Model file for the job. Use its own axes, mm. A direction names the side the tool comes from. Coordinates: 2 decimals unless noted, no trailing zeros. Write each loop counter-clockwise with the first axis right and the second up, starting at its lowest first coordinate (ties: lowest second). Pieces come first, ordered by that corner, then holes. Notation, with made-up numbers: (6.5, -23.75) - (51.5, -23.75) arc R19 cw to (51.5, -7.75) - close; hole circle Ø9 at (46, 34.25). An arc over 180 degrees is marked (long way). Put each result on its own line as item: value. Start each with the question number.
1. Saw through at B-B, the plane z = -21. Write the cut outline in (x, y) (3 decimals), plus the area to 3 significant figures.
2. Which spindle directions (+Z, -Z, +X, -X, +Y, -Y) get a long thin tool onto all of the face, cutting with end or side? Do faces 1 (the face through (9.855, 11.339, -1.565)), 2 (the face through (3.175, 19, -26)). Say none if no direction does.
3. Pull direction Y, two halves, no side cores. Call faces 3 (the face through (2, 19, -47.625)), 4 (the face through (23, 38.1, -18)), 5 (the face through (11.687, 31.793, -1.565)): released by +Y, released by -Y, zero draft, split by the parting line, or undercut.
4. Drop flat-ended pins along their axis: P1, Ø5.5, axis at x = 9.5, y = 20.5, coming from the -Z side (3 decimals); P2, Ø4, axis at y = 14.5, z = -10.5, coming from the -X side. Give the stop position or say it passes through.
5. Drill centre lines: L1, parallel to Y at x = 12.7, z = -1.1; L2, parallel to X at y = 21.5, z = -15 (3 decimals); L3, parallel to Y at x = 24.5, z = -38.1. Where is each one in solid material? Low to high. Write a range as from..to.
6. Saw through at C-C, the plane z = -38.1. Write the cut outline in (x, y) (3 decimals), plus the area to 3 significant figures.
7. Saw through at D-D, the plane y = 18.5. Write the cut outline in (x, z) (3 decimals).
8. Saw through at A-A, the plane x = 12.7. Write the cut outline in (y, z) (3 decimals), plus the area to 3 significant figures.
Autodesk Inventor part; units mm, degrees
ref_plane "YZ Plane" through (0, 0, 0) normal (1, 0, 0) x (0, 1, 0)
ref_plane "XZ Plane" through (0, 0, 0) normal (0, 1, 0) x (-1, 0, 0)
ref_plane "XY Plane" through (0, 0, 0) normal (0, 0, 1) x (1, 0, 0)
sketch "Sketch1" plane through (0, 0, 0) normal (0, 1, 0) x (-1, 0, 0)
  line L0 (0, 0) -> (0, -47.625)
  line L1 (0, -47.625) -> (-3.175, -47.625)
  line L2 (-3.175, -47.625) -> (-3.175, -3.175)
  line L3 (-3.175, -3.175) -> (-22.225, -3.175)
  line L4 (-22.225, -3.175) -> (-22.225, -47.625)
  line L5 (-22.225, -47.625) -> (-25.4, -47.625)
  line L6 (-25.4, -47.625) -> (-25.4, 0)
  line L7 (-25.4, 0) -> (0, 0)
  dimension "d0" = 3.175
  dimension "d1" = 47.625
  dimension "d2" = 3.175
  dimension "d3" = 25.4
  dimension "d4" = 3.175
extrude "Extrusion1" add sketch "Sketch1" along normal blind 38.1
sketch "Sketch2" plane through (25.4, 0, 0) normal (1, 0, 0) x (0, 0, -1)
  line L0 (47.625, 0) -> (47.625, 38.1)
  line L1 (47.625, 0) -> (0, 0)
  point P0 (38.1, 25.4)
  dimension "d7" = 9.525
  dimension "d8" = 25.4
hole "Hole1" at (25.4, 25.4, -38.1) direction (-1, 0, 0) diameter 6.7469 end through all
sketch "Sketch3" plane through (22.225, 0, -3.175) normal (0, 0, -1) x (-1, 0, 0)
  line L0 (-3.175, 0) -> (22.225, 0)
  line L1 (0, 38.1) -> (19.05, 38.1)
  line L2 (22.225, 0) -> (22.225, 38.1)
  line L3 (-3.175, 0) -> (-3.175, 38.1)
  point P0 (9.525, 9.525)
  point P1 (9.525, 28.575)
  point P2 (22.225, 31.75)
  point P3 (-3.175, 31.75)
  dimension "d19" = 9.525
  dimension "d20" = 9.525
  dimension "d21" = 12.7
  dimension "d22" = 12.7
hole "Hole2" at (12.7, 9.525, -3.175) at (12.7, 28.575, -3.175) direction (0, 0, 1) diameter 6.7469 end through all
properties part number "15102898-16-P-0311" material "Aluminum 6061"
Final values:
1. outline: (0, 0) - (3.175, 0) - (3.175, 38.1) - (0, 38.1) - close; (22.225, 0) - (25.4, 0) - (25.4, 38.1) - (22.225, 38.1) - close
1. area: 242 mm²
2. face 1: +Z, -Z
2. face 2: -Z, +Y, -Y
3. face 3: zero draft
3. face 4: released by +Y
3. face 5: undercut
4. P1: stops at z = -3.175
4. P2: stops at x = 0
5. L1: y = 0..6.15, 12.9..25.2, 31.95..38.1
5. L2: x = 0..3.175, 22.225..25.4
5. L3: y = 0..22.03, 28.77..38.1
6. outline: (0, 0) - (3.175, 0) - (3.175, 22.027) - (0, 22.027) - close; (0, 28.773) - (3.175, 28.773) - (3.175, 38.1) - (0, 38.1) - close; (22.225, 0) - (25.4, 0) - (25.4, 22.027) - (22.225, 22.027) - close; (22.225, 28.773) - (25.4, 28.773) - (25.4, 38.1) - (22.225, 38.1) - close
6. area: 199 mm²
7. outline: (0, -47.625) - (3.175, -47.625) - (3.175, -3.175) - (22.225, -3.175) - (22.225, -47.625) - (25.4, -47.625) - (25.4, 0) - (0, 0) - close
8. outline: (0, -3.175) - (6.152, -3.175) - (6.152, 0) - (0, 0) - close; (12.898, -3.175) - (25.202, -3.175) - (25.202, 0) - (12.898, 0) - close; (31.948, -3.175) - (38.1, -3.175) - (38.1, 0) - (31.948, 0) - close
8. area: 78.1 mm²
